```python
from build123d import *

# Parameters (mm, degrees)
SKETCH1_R           = 1.9812
SKETCH1_R_2         = 9.5885
BOSS_EXTRUDE1_DEPTH = 1.5875


with BuildPart() as part:
    # Sketch1 → Boss-Extrude1 (new body)
    with BuildSketch(Plane.XY):
        with BuildLine():
            Line((-156.779774808, 13.544563035), (-37.44917733, 13.544563035))
            ThreePointArc((-37.44917733, 13.544563035), (-30.455296249, 21.578477211), (-39.376058675, 27.398970946))
            Line((-39.376058675, 27.398970946), (-43.090572863, 30.913874067))
            ThreePointArc((-43.090572863, 30.913874067), (-45.816597783, 48.718236551), (-63.74425571, 50.457666506))
            Line((-63.74425571, 50.457666506), (-67.458769898, 53.972569627))
            ThreePointArc((-67.458769898, 53.972569627), (-68.834377223, 59.933132802), (-74.347952883, 62.582867186))
            Line((-74.347952883, 62.582867186), (-119.880999255, 62.582867186))
            ThreePointArc((-119.880999255, 62.582867186), (-125.394574915, 59.933132802), (-126.770182239, 53.972569627))
            Line((-126.770182239, 53.972569627), (-130.484696428, 50.457666506))
            ThreePointArc((-130.484696428, 50.457666506), (-148.412354355, 48.718236551), (-151.138379275, 30.913874067))
            Line((-151.138379275, 30.913874067), (-154.852893463, 27.398970946))
            ThreePointArc((-154.852893463, 27.398970946), (-163.773655888, 21.578477211), (-156.779774808, 13.544563035))
        make_face()
        with Locations(Location((-37.44917733, 20.605763035, 0), (0, 0, 180))):
            Circle(SKETCH1_R, mode=Mode.SUBTRACT)
        with Locations((-138.330387031, 38.06371511)):
            Circle(SKETCH1_R_2, mode=Mode.SUBTRACT)
        with Locations((-119.880999255, 55.521667186)):
            Circle(SKETCH1_R, mode=Mode.SUBTRACT)
        with Locations((-156.779774808, 20.605763035)):
            Circle(SKETCH1_R, mode=Mode.SUBTRACT)
        with Locations(Location((-74.347952883, 55.521667186, 0), (0, 0, 180))):
            Circle(SKETCH1_R, mode=Mode.SUBTRACT)
        with Locations(Location((-55.898565106, 38.06371511, 0), (0, 0, 180))):
            Circle(SKETCH1_R_2, mode=Mode.SUBTRACT)
    extrude(amount=BOSS_EXTRUDE1_DEPTH)


solid = part.part
```
Work out the finished part from the listing and answer in its coordinate system (mm). Coordinates: 2 decimals unless noted, no trailing zeros. Order: outer loops, then holes, each group sorted by start corner. A loop starts at its lowest first (then second) coordinate and runs counter-clockwise, first axis right, second up. Notation, with made-up numbers: M -6.75,-36 L 16.25,-36 A28 cw 16.25,-15 Z; hole C 40.25,88 d7. An arc over 180 degrees is marked long. Use CSV: the item, a comma, the result in double quotes.
1) Section C-C on z = 0.9 is taken. Write down the section's boundary in (x, y).
Worked out:
outline,"M -156.78,13.54 L -37.45,13.54 A7.06 ccw long -39.38,27.4 L -43.09,30.91 A14.67 ccw -63.74,50.46 L -67.46,53.97 A7.06 ccw -74.35,62.58 L -119.88,62.58 A7.06 ccw -126.77,53.97 L -130.48,50.46 A14.67 ccw -151.14,30.91 L -154.85,27.4 A7.06 ccw long Z; hole C -156.78,20.61 d3.96; hole C -138.33,38.06 d19.18; hole C -119.88,55.52 d3.96; hole C -74.35,55.52 d3.96; hole C -55.9,38.06 d19.18; hole C -37.45,20.61 d3.96"
2) Section B-B on y = 44 is taken. Write down the section's boundary in (x, z), plus the area to 3 significant figures.
Worked out:
outline,"M -151.74,0 L -145.86,0 L -145.86,1.59 L -151.74,1.59 Z; M -130.8,0 L -63.43,0 L -63.43,1.59 L -130.8,1.59 Z; M -48.37,0 L -42.48,0 L -42.48,1.59 L -48.37,1.59 Z"
area,"126 mm^2"
3) Section A-A on x = -58 is taken. Write down the section's boundary in (y, z), plus the area to 3 significant figures.
Worked out:
outline,"M 13.54,0 L 28.71,0 L 28.71,1.59 L 13.54,1.59 Z; M 47.42,0 L 52.58,0 L 52.58,1.59 L 47.42,1.59 Z"
area,"32.3 mm^2"
4) Section D-D on x = -134 is taken. Write down the section's boundary in (y, z), plus the area to 3 significant figures.
Worked out:
outline,"M 13.54,0 L 29.51,0 L 29.51,1.59 L 13.54,1.59 Z; M 46.62,0 L 52.08,0 L 52.08,1.59 L 46.62,1.59 Z"
area,"34.0 mm^2"
5) Determine the mould class of faces 1 (the face through (-65.576, 52.191, 0.783)), 2 (the face through (-98, 33, 0)), 3 (the face through (-68.779, 59.864, 0.783)) for opening direction X: released by +X, released by -X, zero draft, split by the parting line, or undercut.
Worked out:
face 1,"undercut"
face 2,"zero draft"
face 3,"released by +X"
6) A flat-ended cylindrical pin translates along its axis: pin 1 Ø8 at (x, y) = (-134, 37) entering from -Z. Find the tip coordinate at first contact, or state that the pin passes through.
Worked out:
pin 1,"passes through"
7) Consider line 1 (X direction, y = 20.5, z = 0.95); line 2 (X direction, y = 33.5, z = 0.7); line 3 (Y direction, x = -56, z = 1.3). Determine where each line is inside the solid, lowest interval first. Write a range as [from, to].
Worked out:
line 1,"x = [-163.84, -158.76], [-154.8, -39.43], [-35.47, -30.39]"
line 2,"x = [-152.27, -146.76], [-129.9, -64.33], [-47.47, -41.96]"
line 3,"y = [13.54, 28.48], [47.65, 52.73]"
